Here's how the part is built. I have some questions about the finished solid (model axes, mm). A direction names the side the tool comes from. Round coordinates to 2 decimals unless told otherwise and drop trailing zeros. Order: outer loops, then holes, each group sorted by start corner. A loop starts at its lowest first (then second) coordinate and runs counter-clockwise, first axis right, second up. Notation, with made-up numbers: (1.5, -0.75) - (41.5, -0.75) arc R23 cw to (41.5, 12.25) - close; hole circle Ø6 at (60, 57). An arc over 180 degrees is marked (long way). Answer as a JSON object with one key per item and string values.
Autodesk Inventor part; units mm, degrees
ref_plane "YZ Plane" through (0, 0, 0) normal (1, 0, 0) x (0, 1, 0)
ref_plane "XZ Plane" through (0, 0, 0) normal (0, 1, 0) x (-1, 0, 0)
ref_plane "XY Plane" through (0, 0, 0) normal (0, 0, 1) x (1, 0, 0)
sketch "Sketch1" plane through (0, 0, 0) normal (0, 1, 0) x (-1, 0, 0)
  line L0 (0, 0) -> (30.1498, 0)
  line L1 (30.1498, 0) -> (30.1498, -30.1498)
  line L2 (30.1498, -30.1498) -> (0, -30.1498)
  line L3 (0, -30.1498) -> (0, 0)
  dimension "d0" = 30.1498
  dimension "d1" = 30.1498
extrude "Extrusion1" add sketch "Sketch1" along normal blind 9.652
sketch "Sketch3" plane through (0, 9.652, 0) normal (0, 1, 0) x (1, 0, 0)
  line L0 (-30.1498, 0) -> (0, 0)
  line L1 (0, 0) -> (0, 30.1498)
  line L2 (0, 30.1498) -> (-30.1498, 30.1498)
  line L3 (-30.1498, 30.1498) -> (-30.1498, 0)
  line L4 (-30.1498, 0) -> (0, 0)
  line L5 (-15.0749, 0) -> (-28.7909, 0)
  line L6 (-30.1498, 30.1498) -> (-30.1498, 0)
  line L7 (-30.1498, 15.0749) -> (-30.1498, 1.3589)
  line L8 (-30.1498, 1.3589) -> (-30.1498, 3.0861)
  line L9 (-30.1498, 3.0861) -> (-27.0637, 3.0861)
  line L10 (-28.7909, 0) -> (-27.0637, 0)
  line L11 (-27.0637, 0) -> (-27.0637, 3.0861)
  circle A0 centre (-27.0637, 3.0861) radius 1.7272
  line L12 (-15.0749, 0) -> (-15.0749, 4.3585)
  line L13 (-30.1498, 15.0749) -> (-29.1171, 15.0749)
  circle A1 centre (-3.0861, 3.0861) radius 1.7272
  line L14 (0, 15.0749) -> (-1.0327, 15.0749)
  circle A2 centre (-27.0637, 27.0637) radius 1.7272
  circle A3 centre (-3.0861, 27.0637) radius 1.7272
  dimension "d9" = 13.716
  dimension "d10" = 13.716
  dimension "d11" = 1.7272
  dimension "d12" = 1.7272
  dimension "d13" = 3.4544
extrude "Extrusion3" cut sketch "Sketch3" against normal blind 30.48 contours A0 L9 L11 | L11 L9 A0 | A1 | A2 | A3
sketch "Sketch4" plane through (0, 0, 0) normal (1, 0, 0) x (0, 0, -1)
  line L0 (4.8133, 9.652) -> (4.8133, 0)
  line L1 (1.3589, 9.652) -> (1.3589, 0)
  line L2 (4.8133, 4.826) -> (9.6393, 4.826)
  circle A0 centre (4.9912, 4.826) radius 2.921
  line L3 (30.1498, 0) -> (0, 0)
  line L4 (30.1498, 0) -> (30.1498, 9.652)
  line L5 (0, 9.652) -> (30.1498, 9.652)
  line L6 (0, 0) -> (0, 9.652)
  line L7 (0, 4.826) -> (-2.921, 4.826)
  circle A1 centre (-2.921, 4.826) radius 2.921
  line L8 (0, 0) -> (-7.747, 0)
  line L9 (-7.747, 0) -> (-7.747, 9.652)
  line L10 (-7.747, 9.652) -> (0, 9.652)
  line L11 (0, 9.652) -> (0, 0)
  dimension "d16" = 4.826
  dimension "d18" = 2.921
  dimension "d19" = 7.747
extrude "Extrusion4" add sketch "Sketch4" against normal up to surface (30.1498 mm away) contours L6 L8 L9 L10
sketch "Sketch5" plane through (0, 9.652, 0) normal (0, 1, 0) x (1, 0, 0)
  circle A0 centre (-3.0861, 27.0637) radius 1.7272
  circle A1 centre (-3.0861, 3.0861) radius 1.7272
  circle A2 centre (-27.0637, 3.0861) radius 1.7272
  circle A3 centre (-27.0637, 27.0637) radius 1.7272
  line L0 (0, 30.1498) -> (0, -7.747)
  line L1 (0, 30.1498) -> (-30.1498, 30.1498)
  line L2 (-30.1498, 30.1498) -> (-30.1498, -7.747)
  line L3 (0, -7.747) -> (-30.1498, -7.747)
  circle A4 centre (-27.0637, 27.0637) radius 1.7272
  circle A5 centre (-27.0637, 22.2631) radius 1.7272
  circle A6 centre (-27.0637, 17.4625) radius 1.7272
  circle A7 centre (-27.0637, 12.6619) radius 1.7272
  circle A8 centre (-27.0637, 7.8613) radius 1.7272
  circle A9 centre (-27.0637, 3.0607) radius 1.7272
  circle A10 centre (-22.2631, 27.0637) radius 1.7272
  circle A11 centre (-22.2631, 22.2631) radius 1.7272
  circle A12 centre (-22.2631, 17.4625) radius 1.7272
  circle A13 centre (-22.2631, 12.6619) radius 1.7272
  circle A14 centre (-22.2631, 7.8613) radius 1.7272
  circle A15 centre (-22.2631, 3.0607) radius 1.7272
  circle A16 centre (-17.4625, 27.0637) radius 1.7272
  circle A17 centre (-17.4625, 22.2631) radius 1.7272
  circle A18 centre (-17.4625, 17.4625) radius 1.7272
  circle A19 centre (-17.4625, 12.6619) radius 1.7272
  circle A20 centre (-17.4625, 7.8613) radius 1.7272
  circle A21 centre (-17.4625, 3.0607) radius 1.7272
  circle A22 centre (-12.6619, 27.0637) radius 1.7272
  circle A23 centre (-12.6619, 22.2631) radius 1.7272
  circle A24 centre (-12.6619, 17.4625) radius 1.7272
  circle A25 centre (-12.6619, 12.6619) radius 1.7272
  circle A26 centre (-12.6619, 7.8613) radius 1.7272
  circle A27 centre (-12.6619, 3.0607) radius 1.7272
  circle A28 centre (-7.8613, 27.0637) radius 1.7272
  circle A29 centre (-7.8613, 22.2631) radius 1.7272
  circle A30 centre (-7.8613, 17.4625) radius 1.7272
  circle A31 centre (-7.8613, 12.6619) radius 1.7272
  circle A32 centre (-7.8613, 7.8613) radius 1.7272
  circle A33 centre (-7.8613, 3.0607) radius 1.7272
  circle A34 centre (-3.0607, 27.0637) radius 1.7272
  circle A35 centre (-3.0607, 22.2631) radius 1.7272
  circle A36 centre (-3.0607, 17.4625) radius 1.7272
  circle A37 centre (-3.0607, 12.6619) radius 1.7272
  circle A38 centre (-3.0607, 7.8613) radius 1.7272
  circle A39 centre (-3.0607, 3.0607) radius 1.7272
  point P0 (0, 0)
  dimension "d24" = 4.8006
  dimension "d27" = 4.8006
extrude "Extrusion5" cut sketch "Sketch5" against normal blind 30.48 contours A5 | A6 | A7 | A8 | A10 | A11 | A12 | A13 | A14 | A15 | A16 | A17 | A18 | A19 | A20 | A21 | A22 | A23 | A24 | A25 | A26 | A27 | A28 | A29 | A30 | A31 | A32 | A33 | A35 | A36 | A37 | A38
sketch "Sketch6" plane through (0, 0, -30.1498) normal (1, 0, 0) x (0, 0, -1)
  circle A0 centre (-33.0708, 4.826) radius 2.921
  line L0 (0, 9.652) -> (-37.8968, 9.652)
  line L1 (-37.8968, 9.652) -> (-37.8968, 0)
  line L2 (-37.8968, 0) -> (0, 0)
  line L3 (0, 0) -> (0, 9.652)
  line L4 (-24.0157, 9.652) -> (-24.0157, 0)
  line L5 (-25.3365, 9.652) -> (-25.3365, 0)
  line L6 (-25.3365, 4.826) -> (-24.0157, 4.826)
  line L7 (-24.6761, 4.826) -> (-25.3365, 4.826)
  line L8 (-28.7909, 9.652) -> (-28.7909, 0)
  line L9 (-25.0063, 4.826) -> (-24.1173, 4.826)
  circle A1 centre (-24.1173, 4.826) radius 0.889
  point P0 (-30.1498, 0)
  dimension "d33" = 0.889
  dimension "d34" = 1.778
sketch "Sketch7" plane through (0, 9.652, 0) normal (0, 1, 0) x (1, 0, 0)
  circle A0 centre (-3.0607, 7.8613) radius 1.7272
  point P0 (0, 0)
extrude "Extrusion6" add sketch "Sketch7" against normal blind 9.652
extrude "Extrusion7" cut sketch "Sketch6" against normal blind 6.35 contours A1 L4 | L4 L6 A1 | L4 A1 L6
sketch "Sketch8" plane through (0, 0, -30.1498) normal (1, 0, 0) x (0, 0, -1)
  circle A0 centre (-24.1173, 4.826) radius 0.889
  circle A1 centre (-33.0708, 4.826) radius 2.921
  line L0 (0, 9.652) -> (-37.8968, 9.652)
  line L1 (-37.8968, 9.652) -> (-37.8968, 0)
  line L2 (-37.8968, 0) -> (0, 0)
  line L3 (0, 0) -> (0, 9.652)
  line L4 (0, 0) -> (0, 9.652)
  line L5 (0, 4.826) -> (0, 0)
  line L6 (-1.3589, 0) -> (-4.8133, 0)
  line L7 (0, 4.826) -> (4.826, 4.826)
  circle A2 centre (4.826, 4.826) radius 4.826
  line L8 (0, 9.652) -> (4.826, 9.652)
  line L9 (4.826, 0) -> (0, 0)
  point P0 (-30.1498, 0)
  dimension "d39" = 4.826
  dimension "d40" = 4.826
extrude "Extrusion8" add sketch "Sketch8" against normal up to surface (30.1498 mm away) contours L8 A2 L3 | A2 L9 L3 | A2
sketch "Sketch9" plane through (0, 0, 7.747) normal (1, 0, 0) x (0, 0, -1)
  circle A0 centre (13.7795, 4.826) radius 0.889
  circle A1 centre (4.826, 4.826) radius 2.921
  line L0 (42.7228, 9.652) -> (0, 9.652)
  line L1 (0, 9.652) -> (0, 0)
  line L2 (0, 0) -> (42.7228, 0)
  arc A2 (42.7228, 0) -> (42.7228, 9.652) centre (42.7228, 4.826) ccw
  circle A3 centre (42.7228, 4.826) radius 1.4986
  point P0 (7.747, 0)
  dimension "d43" = 2.9972
extrude "Extrusion9" cut sketch "Sketch9" against normal through all contours A3
sketch "Sketch10" plane through (0, 9.652, 0) normal (0, 1, 0) x (1, 0, 0)
  circle A0 centre (-3.0607, 12.6619) radius 1.7272
  circle A1 centre (-3.0607, 22.2631) radius 1.7272
  circle A2 centre (-7.8613, 7.8613) radius 1.7272
  circle A3 centre (-7.8613, 17.4625) radius 1.7272
  circle A4 centre (-7.8613, 27.0637) radius 1.7272
  circle A5 centre (-12.6619, 7.8613) radius 1.7272
  circle A6 centre (-12.6619, 17.4625) radius 1.7272
  circle A7 centre (-12.6619, 27.0637) radius 1.7272
  circle A8 centre (-17.4625, 7.8613) radius 1.7272
  circle A9 centre (-17.4625, 17.4625) radius 1.7272
  circle A10 centre (-17.4625, 27.0637) radius 1.7272
  circle A11 centre (-22.2631, 7.8613) radius 1.7272
  circle A12 centre (-22.2631, 17.4625) radius 1.7272
  circle A13 centre (-22.2631, 27.0637) radius 1.7272
  circle A14 centre (-27.0637, 12.6619) radius 1.7272
  circle A15 centre (-27.0637, 22.2631) radius 1.7272
  circle A16 centre (-27.0637, 17.4625) radius 1.7272
  circle A17 centre (-27.0637, 7.8613) radius 1.7272
  circle A18 centre (-22.2631, 22.2631) radius 1.7272
  circle A19 centre (-22.2631, 12.6619) radius 1.7272
  circle A20 centre (-22.2631, 3.0607) radius 1.7272
  circle A21 centre (-17.4625, 22.2631) radius 1.7272
  circle A22 centre (-17.4625, 12.6619) radius 1.7272
  circle A23 centre (-17.4625, 3.0607) radius 1.7272
  circle A24 centre (-12.6619, 22.2631) radius 1.7272
  circle A25 centre (-12.6619, 12.6619) radius 1.7272
  circle A26 centre (-12.6619, 3.0607) radius 1.7272
  circle A27 centre (-7.8613, 22.2631) radius 1.7272
  circle A28 centre (-7.8613, 12.6619) radius 1.7272
  circle A29 centre (-7.8613, 3.0607) radius 1.7272
  circle A30 centre (-3.0607, 17.4625) radius 1.7272
  circle A31 centre (-3.0861, 27.0637) radius 1.7272
  circle A32 centre (-3.0861, 3.0861) radius 1.7272
  circle A33 centre (-27.0637, 3.0861) radius 1.7272
  circle A34 centre (-27.0637, 27.0637) radius 1.7272
  line L0 (0, 34.9758) -> (0, -7.747)
  line L1 (0, 34.9758) -> (-30.1498, 34.9758) construction
  line L2 (-30.1498, 34.9758) -> (-30.1498, -7.747)
  line L3 (0, -7.747) -> (-30.1498, -7.747)
  line L4 (0, 36.4744) -> (-30.1498, 36.4744) construction
  line L5 (-30.1498, 34.9758) -> (-30.1498, 34.9758)
  line L6 (0, 34.9758) -> (-30.1498, 34.9758) construction
  line L7 (0, 34.9758) -> (0, 34.9758)
  line L8 (0, 34.9758) -> (-30.1498, 34.9758)
  line L9 (-30.1498, 34.9758) -> (-30.1498, 39.8018)
  line L10 (0, 34.9758) -> (0, 39.8018)
  line L11 (0, 33.4772) -> (-30.1498, 33.4772) construction
  line L12 (-30.1498, 34.9758) -> (-30.1498, -7.747)
  line L13 (-30.1498, 30.076) -> (0, 30.076)
  line L14 (0, 30.076) -> (0, 39.8018)
  line L15 (-30.1498, 39.8018) -> (-30.1498, 30.076)
  line L16 (-15.0749, 39.8018) -> (-15.0749, 30.076)
  line L17 (0, 34.9758) -> (-30.1498, 34.9758)
  line L18 (-15.0749, 34.9758) -> (-30.1498, 34.9758) construction
  line L19 (-30.1498, 34.9758) -> (-22.6123, 34.9758)
  line L20 (-22.6123, 34.9758) -> (-22.6123, 39.8018)
  line L21 (-22.6123, 34.9758) -> (-22.6123, 30.076)
  line L22 (0, 34.9758) -> (-7.5374, 34.9758)
  line L23 (-7.5374, 39.8018) -> (-7.5374, 30.076)
  line L24 (-26.3811, 30.076) -> (-26.3811, 39.8018)
  line L25 (-22.6123, 30.076) -> (-15.0749, 30.076)
  line L26 (-18.8436, 30.076) -> (-18.8436, 39.8018)
  line L27 (-7.5374, 30.076) -> (-15.0749, 30.076)
  line L28 (-11.3062, 30.076) -> (-11.3062, 39.8018)
  line L29 (0, 30.076) -> (-7.5374, 30.076)
  line L30 (-3.7687, 30.076) -> (-3.7687, 39.8018)
  line L31 (-3.7687, 30.076) -> (-7.5374, 30.076)
  line L32 (-7.5374, 30.076) -> (-7.5374, 39.8018)
  line L33 (-7.5374, 39.8018) -> (-3.7687, 39.8018)
  line L34 (-3.7687, 39.8018) -> (-3.7687, 30.076)
  line L35 (-11.3062, 30.076) -> (-15.0749, 30.076)
  line L36 (-15.0749, 30.076) -> (-15.0749, 39.8018)
  line L37 (-15.0749, 39.8018) -> (-11.3062, 39.8018)
  line L38 (-11.3062, 39.8018) -> (-11.3062, 30.076)
  line L39 (-18.8436, 30.076) -> (-22.6123, 30.076)
  line L40 (-22.6123, 30.076) -> (-22.6123, 39.8018)
  line L41 (-18.8436, 39.8018) -> (-18.8436, 30.076)
  line L42 (-22.6123, 30.076) -> (-26.3811, 30.076)
  line L43 (-26.3811, 30.076) -> (-26.3811, 39.8018)
  line L44 (-26.3811, 39.8018) -> (-22.6123, 39.8018)
  line L45 (-22.6123, 39.8018) -> (-22.6123, 30.076)
  line L46 (-3.7687, 30.076) -> (-7.5374, 30.076)
  line L47 (-7.5374, 30.076) -> (-7.5374, 39.8018)
  line L48 (-7.5374, 39.8018) -> (-3.7687, 39.8018)
  line L49 (-3.7687, 39.8018) -> (-3.7687, 30.076)
  line L50 (-11.3062, 30.076) -> (-18.8436, 30.076)
  line L51 (-18.8436, 30.076) -> (-18.8436, 39.8018)
  line L52 (-18.8436, 39.8018) -> (-11.3062, 39.8018)
  line L53 (-11.3062, 39.8018) -> (-11.3062, 30.076)
  point P0 (0, 0)
extrude "Extrusion10" cut sketch "Sketch10" against normal through all contours L30 L13 L23 L8 | L8 L23 L33 L30 | L28 L13 L16 L8 | L8 L16 L37 L28 | L16 L13 L26 L8 | L8 L26 L52 L16 | L24 L8 L21 L13 | L24 L44 L20 L8
properties part number "left wing" material "Aluminum 6061"
1. Imagine slicing it at D-D (z = -18). List the corners of the cut face in (x, y) for me, plus the area to 3 significant figures.
Responses:
{"outline": "(-30.15, 0) - (-28.71, 0) - (-28.71, 9.65) - (-30.15, 9.65) - close; (-25.42, 0) - (-23.9, 0) - (-23.9, 9.65) - (-25.42, 9.65) - close; (-20.62, 0) - (-19.1, 0) - (-19.1, 9.65) - (-20.62, 9.65) - close; (-15.82, 0) - (-14.3, 0) - (-14.3, 9.65) - (-15.82, 9.65) - close; (-11.02, 0) - (-9.5, 0) - (-9.5, 9.65) - (-11.02, 9.65) - close; (-6.22, 0) - (-4.7, 0) - (-4.7, 9.65) - (-6.22, 9.65) - close; (-1.42, 0) - (0, 0) - (0, 9.65) - (-1.42, 9.65) - close", "area": "101 mm2"}
2. Thinking about a two-plate mould opening in X: for faces 1 (the face through (-6, 5, -30.076)), 2 (the face through (-9.4, 4.7, -39.8)), which applies, pulls with the +X half, pulls with the -X half, needs draft (parallel to the pull), parting line crosses it, or undercut?
Responses:
{"face 1": "undercut", "face 2": "needs draft"}
3. If I drill on L1, parallel to X at y = 1.75, z = -33; L2, parallel to X at y = 2.5, z = -7; L3, parallel to Z at x = -1, y = 4.5, over which ranges is the centre line in solid material (lowest first)? Write a range as [from, to].
Responses:
{"L1": "[-30.15, -26.38], [-22.61, -18.84], [-11.31, -7.54], [-3.77, 0]", "L2": "[-30.15, -28.56], [-25.57, -23.76], [-20.77, -18.96], [-15.97, -14.16], [-11.16, -9.36], [-6.36, 0]", "L3": "[-39.79, -36.44], [-33.51, -6.86], [-5.21, 0.02], [5.82, 7.75]"}
4. Imagine slicing it at A-A (x = -21). Give the number of separate pieces and of enclosed holes in the cut face, plus the area to 3 significant figures.
Responses:
{"separate pieces": "7", "enclosed holes": "2", "area": "279 mm2"}
5. For faces 3 (the face through (-11.7, 4.9, -23.7)), 4 (the face through (-3.769, 6, -33.8)), which set-ups out of +Z, -Z, +X, -X, +Y, -Y let a thin tool reach every point of the face, with its end or its side?
Responses:
{"face 3": "+Y, -Y", "face 4": "-Z, +Y, -Y"}
